Source: CAD feature listing. Evaluate the final solid. Frame: model axes, mm. A direction names the side the tool comes from. Give positions to 0.01 mm unless a question says otherwise; leave off trailing zeros. Order: outer loops, then holes, each group sorted by start corner. A loop starts at its lowest first (then second) coordinate and runs counter-clockwise, first axis right, second up. Notation, with made-up numbers: M 1,62 L 27,62 A7 ccw 27,69 Z; hole C 66,-18 d1. An arc over 180 degrees is marked long. Use CSV: the item, a comma, the result in double quotes. Start each with the question number.
1. Section query A-A, the plane z = 0. Return the cut outline in (x, y).
2. Line query: line 1 along X through (y, z) = (2, 0); line 2 along Z through (x, y) = (0, 2.25); line 3 along Y through (x, z) = (-20, -16). Output: solid intervals per line, ascending. Write a range as [from, to].
3. Mould query, pull axis Z, two halves, no side actions, for faces 1 (the cylindrical face through (-1.38, 3.13, 6.2)), 2 (the flat face through (1, 81, 31.75)), 3 (the flat face through (-1, 158.75, 44)). Classes: released by +Z, released by -Z, zero draft, split by the parting line, or undercut.
4. Section query B-B, the plane x = 0. Return the cut outline in (y, z).
5. Reachability of faces 4 (the cylindrical face through (1.61, 78.26, 41.2)), 5 (the flat face through (-1, 6.35, -13)) from +Z, -Z, +X, -X, +Y, -Y: full face, straight path, thin tool, end or side. Return the list, or none.
6. Section query D-D, the plane z = -38.1. Return the cut outline in (x, y), plus the area to 3 significant figures.
7. Pin query (flat end, axial travel): P1, Ø4, axis at x = 0, z = -38.1, coming from the +Y side; P2, Ø2, axis at x = -39.5, y = 129, coming from the -Z side; P3, Ø4, axis at x = -21, z = -36, coming from the -Y side; P4, Ø8, axis at x = -25.4, z = 0, coming from the +Y side. Return the tip coordinate at first contact, or that it passes through.
from build123d import *

# Parameters (mm, degrees)
SKETCH1_R                  = 57.15
SKETCH1_R_2                = 6.35
SKETCH1_R_3                = 3.4925
BOSS_EXTRUDE1_DEPTH        = 6.35
F_8_0_199_DIAMETER_HOLE1_D = 5.0546
SKETCH6_R                  = 3.4925
BOSS_EXTRUDE3_DEPTH        = 152.4


with BuildPart() as part:
    # Sketch1 → Boss-Extrude1 (new body)
    with BuildSketch(Plane(origin=(0, 0, 0), x_dir=(1, 0, 0), z_dir=(0, 1, 0))):
        Circle(SKETCH1_R)
        Circle(SKETCH1_R_2, mode=Mode.SUBTRACT)
        with Locations((0, 38.1)):
            Circle(SKETCH1_R_3, mode=Mode.SUBTRACT)
        with Locations((0, -38.1)):
            Circle(SKETCH1_R_3, mode=Mode.SUBTRACT)
    extrude(amount=BOSS_EXTRUDE1_DEPTH)

    # #8 (0.199) Diameter Hole1 (through all)
    with Locations(Plane(origin=(-25.4, 6.35, 0), x_dir=(0, 0, 1), z_dir=(0, 1, 0))):
        with Locations((0, 0), (0, 50.8)):
            Hole(F_8_0_199_DIAMETER_HOLE1_D / 2)

    # Sketch6 → Boss-Extrude3 (add)
    with BuildSketch(Plane(origin=(0, 6.35, 0), x_dir=(1, 0, 0), z_dir=(0, 1, 0))):
        with BuildLine():
            Line((47.519048812, -31.75), (-47.519048812, -31.75))
            ThreePointArc((-47.519048812, -31.75), (0, -57.15), (47.519048812, -31.75))
        make_face()
        with Locations((0, -38.1)):
            Circle(SKETCH6_R, mode=Mode.SUBTRACT)
    extrude(amount=BOSS_EXTRUDE3_DEPTH)


solid = part.part
Result set:
1,outline,"M -57.15,0 L -27.93,0 L -27.93,6.35 L -57.15,6.35 Z; M -22.87,0 L -6.35,0 L -6.35,6.35 L -22.87,6.35 Z; M 6.35,0 L 22.87,0 L 22.87,6.35 L 6.35,6.35 Z; M 27.93,0 L 57.15,0 L 57.15,6.35 L 27.93,6.35 Z"
2,line 1,"[-57.15, -27.93], [-22.87, -6.35], [6.35, 22.87], [27.93, 57.15]"
2,line 2,"[-57.15, -41.59], [-34.61, -6.35], [6.35, 34.61], [41.59, 57.15]"
2,line 3,"[0, 6.35]"
3,face 1,"undercut"
3,face 2,"released by -Z"
3,face 3,"zero draft"
4,outline,"M 0,-57.15 L 6.35,-57.15 L 6.35,-41.59 L 0,-41.59 Z; M 0,-34.61 L 6.35,-34.61 L 6.35,-6.35 L 0,-6.35 Z; M 0,6.35 L 6.35,6.35 L 6.35,31.75 L 158.75,31.75 L 158.75,34.61 L 0,34.61 Z; M 0,41.59 L 158.75,41.59 L 158.75,57.15 L 0,57.15 Z"
5,face 4,"+Y, -Y"
5,face 5,"-Z, +X, -X, +Y"
6,outline,"M -42.6,0 L -3.49,0 L -3.49,6.35 L -42.6,6.35 Z; M 3.49,0 L 42.6,0 L 42.6,6.35 L 3.49,6.35 Z"
6,area,"497 mm2"
7,P1,"through"
7,P2,"z = 31.75"
7,P3,"y = 0"
7,P4,"y = 6.35"
